```python
from build123d import *

# Parameters (mm, degrees)
BOSS_EXTRUDE1_DEPTH              = 320.675
BOSS_EXTRUDE1_DEPTH_BACK         = 320.675
SKETCH3_W                        = 50.8
SKETCH3_H                        = 25.4
SKETCH3_W_2                      = 44.45
SKETCH3_H_2                      = 19.05
CUT_EXTRUDE1_DEPTH               = 323.680609311
CUT_EXTRUDE1_DEPTH_BACK          = 323.680609311
SKETCH8_R                        = 14.2875
CUT_EXTRUDE2_DEPTH               = 323.680609311
F_10_CLEARANCE_HOLE1_D           = 4.9784
F_10_CLEARANCE_HOLE1_DEPTH       = 5.08
F_10_CLEARANCE_HOLE1_TIP         = 1.495662253
F_10_CLEARANCE_HOLE2_D           = 4.9784
F_10_CLEARANCE_HOLE3_D           = 4.9784
TAP_DRILL_FOR_8_32_TAP1_D        = 3.4544
F_10_CLEARANCE_HOLE4_AT_2_COUNT  = 2
F_10_CLEARANCE_HOLE4_AT_2_PITCH  = 21.6408
F_10_CLEARANCE_HOLE4_AT_3_COUNT  = 2
F_10_CLEARANCE_HOLE4_AT_3_PITCH  = 32.224022105
F_10_CLEARANCE_HOLE4_AT_4_COUNT  = 2
F_10_CLEARANCE_HOLE4_AT_4_PITCH  = 23.876
F_10_CLEARANCE_HOLE4_AT_5_COUNT  = 2
F_10_CLEARANCE_HOLE4_AT_5_PITCH  = 245.0465
F_10_CLEARANCE_HOLE4_AT_6_COUNT  = 2
F_10_CLEARANCE_HOLE4_AT_6_PITCH  = 246.000226396
F_10_CLEARANCE_HOLE4_AT_7_COUNT  = 2
F_10_CLEARANCE_HOLE4_AT_7_PITCH  = 268.9225
F_10_CLEARANCE_HOLE4_AT_8_COUNT  = 2
F_10_CLEARANCE_HOLE4_AT_8_PITCH  = 269.79183685
F_10_0_1935_DIAMETER_HOLE1_D     = 4.9149
F_10_0_1935_DIAMETER_HOLE1_DEPTH = 3.302
F_10_0_1935_DIAMETER_HOLE1_TIP   = 1.476584928
CUT_EXTRUDE3_DEPTH               = 323.680609311


with BuildPart() as part:
    # Sketch3 → Boss-Extrude1 (new, two sides: drawn at the far end of the back side and taken through both)
    with BuildSketch(Plane.XY.offset(-BOSS_EXTRUDE1_DEPTH_BACK)):
        Rectangle(SKETCH3_W, SKETCH3_H)
        Rectangle(SKETCH3_W_2, SKETCH3_H_2, mode=Mode.SUBTRACT)
    extrude(amount=BOSS_EXTRUDE1_DEPTH + BOSS_EXTRUDE1_DEPTH_BACK)

    # Sketch4 → Cut-Extrude1 (cut, two sides: drawn at the far end of the back side and taken through both)
    with BuildSketch(Plane(origin=(0, 12.7, 0), x_dir=(1, 0, 0), z_dir=(0, 1, 0)).offset(-CUT_EXTRUDE1_DEPTH_BACK)):
        Polygon((1322.117470931, -320.675), (25.4, -320.675), (-25.4, -320.675), (25.4, -305.627354456), (1268.718301677, 62.660305034), (3837.350959621, 420.474595165), (3890.750128875, 37.139290131), align=None)
    extrude(amount=CUT_EXTRUDE1_DEPTH + CUT_EXTRUDE1_DEPTH_BACK, mode=Mode.SUBTRACT)

    # Sketch8 → Cut-Extrude2 (cut, through all)
    with BuildSketch(Plane(origin=(0, 12.7, 0), x_dir=(1, 0, 0), z_dir=(0, 1, 0))):
        with Locations(Location((0, 266.954, 0), (0, 0, 180))):
            Circle(SKETCH8_R)
    extrude(amount=-CUT_EXTRUDE2_DEPTH, mode=Mode.SUBTRACT)

    # #10 Clearance Hole1
    with Locations(Plane(origin=(0, 12.7, 0), x_dir=(1, 0, 0), z_dir=(0, 1, 0))):
        with Locations((-12.7762, -284.753033923), (12.6238, -284.753033923), (12.6238, -301.263033923), (-12.7762, -301.263033923)):
            Hole(F_10_CLEARANCE_HOLE1_D / 2, depth=F_10_CLEARANCE_HOLE1_DEPTH)
            with Locations((0, 0, -(F_10_CLEARANCE_HOLE1_DEPTH + F_10_CLEARANCE_HOLE1_TIP / 2))):  # 118° drill point
                Cone(0, F_10_CLEARANCE_HOLE1_D / 2, F_10_CLEARANCE_HOLE1_TIP, mode=Mode.SUBTRACT)

    # #10 Clearance Hole2 (through all)
    with Locations(Plane(origin=(25.4, 0, 0), x_dir=(0, 0, -1), z_dir=(1, 0, 0))):
        with Locations((3.429, -6.35), (28.829, -6.35), (54.229, -6.35), (79.629, -6.35), (105.029, -6.35), (-288.925, -6.35), (-263.525, -6.35), (-238.126133061, -6.35)):
            Hole(F_10_CLEARANCE_HOLE2_D / 2)

    # #10 Clearance Hole3 (through all)
    with Locations(Plane(origin=(25.4, 0, 0), x_dir=(0, 0, -1), z_dir=(1, 0, 0))):
        with Locations((295.275, -6.388229415), (314.325, -6.35)):
            Hole(F_10_CLEARANCE_HOLE3_D / 2)

    # Tap Drill for #8-32 Tap1 (through all)
    with Locations(Plane(origin=(0, -12.7, 0), x_dir=(-1, 0, 0), z_dir=(0, -1, 0))):
        with Locations((-12.751963692, 254.202036308)):
            Hole(TAP_DRILL_FOR_8_32_TAP1_D / 2)

    # Sketch21 → #10 Clearance Hole4 (revolve, cut)
    with BuildSketch(Plane(origin=(11.845144988, -12.7, 30.44825), x_dir=(0, 0, -1), z_dir=(1, 0, 0))):
        Polygon((0, 0), (0, 25.4), (5.2197, 25.4), (2.4892, 22.258919064), (2.4892, 0), align=None)
    f_10_clearance_hole4 = revolve(axis=Axis((11.845144988, -19.05, 30.44825), (0, 1, 0)), mode=Mode.SUBTRACT)

    # #10 Clearance Hole4 at 2: #10 Clearance Hole4 ×2
    with Locations(*[(-i * F_10_CLEARANCE_HOLE4_AT_2_PITCH, 0, 0) for i in range(1, F_10_CLEARANCE_HOLE4_AT_2_COUNT)]):
        add(f_10_clearance_hole4, mode=Mode.SUBTRACT)

    # #10 Clearance Hole4 at 3: #10 Clearance Hole4 ×2
    with Locations(*[Vector(-0.6715735214342001, 0, 0.7409379227090944) * (i * F_10_CLEARANCE_HOLE4_AT_3_PITCH) for i in range(1, F_10_CLEARANCE_HOLE4_AT_3_COUNT)]):
        add(f_10_clearance_hole4, mode=Mode.SUBTRACT)

    # #10 Clearance Hole4 at 4: #10 Clearance Hole4 ×2
    with Locations(*[(0, 0, i * F_10_CLEARANCE_HOLE4_AT_4_PITCH) for i in range(1, F_10_CLEARANCE_HOLE4_AT_4_COUNT)]):
        add(f_10_clearance_hole4, mode=Mode.SUBTRACT)

    # #10 Clearance Hole4 at 5: #10 Clearance Hole4 ×2
    with Locations(*[(0, 0, -i * F_10_CLEARANCE_HOLE4_AT_5_PITCH) for i in range(1, F_10_CLEARANCE_HOLE4_AT_5_COUNT)]):
        add(f_10_clearance_hole4, mode=Mode.SUBTRACT)

    # #10 Clearance Hole4 at 6: #10 Clearance Hole4 ×2
    with Locations(*[Vector(-0.08797065074713521, 0, -0.9961230669988149) * (i * F_10_CLEARANCE_HOLE4_AT_6_PITCH) for i in range(1, F_10_CLEARANCE_HOLE4_AT_6_COUNT)]):
        add(f_10_clearance_hole4, mode=Mode.SUBTRACT)

    # #10 Clearance Hole4 at 7: #10 Clearance Hole4 ×2
    with Locations(*[(0, 0, -i * F_10_CLEARANCE_HOLE4_AT_7_PITCH) for i in range(1, F_10_CLEARANCE_HOLE4_AT_7_COUNT)]):
        add(f_10_clearance_hole4, mode=Mode.SUBTRACT)

    # #10 Clearance Hole4 at 8: #10 Clearance Hole4 ×2
    with Locations(*[Vector(-0.08021295326304817, 0, -0.9967777496156403) * (i * F_10_CLEARANCE_HOLE4_AT_8_PITCH) for i in range(1, F_10_CLEARANCE_HOLE4_AT_8_COUNT)]):
        add(f_10_clearance_hole4, mode=Mode.SUBTRACT)

    # #10 (0.1935) Diameter Hole1
    with Locations(Plane(origin=(25.4, 0, 0), x_dir=(0, 0, -1), z_dir=(1, 0, 0))):
        with Locations((269.875, -6.35)):
            Hole(F_10_0_1935_DIAMETER_HOLE1_D / 2, depth=F_10_0_1935_DIAMETER_HOLE1_DEPTH)
            with Locations((0, 0, -(F_10_0_1935_DIAMETER_HOLE1_DEPTH + F_10_0_1935_DIAMETER_HOLE1_TIP / 2))):  # 118° drill point
                Cone(0, F_10_0_1935_DIAMETER_HOLE1_D / 2, F_10_0_1935_DIAMETER_HOLE1_TIP, mode=Mode.SUBTRACT)

    # Sketch24 → Cut-Extrude3 (cut, through all)
    with BuildSketch(Plane.XZ.offset(12.7)):
        with BuildLine():
            Line((-5.356640498, 314.737886431), (-17.533651131, 318.344881309))
            Line((-17.533651131, 318.344881309), (-18.255050107, 315.909479182))
            ThreePointArc((-18.255050107, 315.909479182), (-13.970042229, 308.017476427), (-6.078039474, 312.302484305))
            Line((-6.078039474, 312.302484305), (-5.356640498, 314.737886431))
        make_face()
    extrude(amount=-CUT_EXTRUDE3_DEPTH, mode=Mode.SUBTRACT)


solid = part.part
```
Read the model definition and answer for the solid it produces. Units are mm, in the model's axes. A direction names the side the tool comes from. Coordinates: 2 decimals unless noted, no trailing zeros. Loops run counter-clockwise (first coordinate to the right, second up) from the corner with the lowest first, then second, coordinate; pieces in that order, holes last. Notation, with made-up numbers: (87.25, 35.25) -> (105.25, 35.25) arc R13 ccw to (105.25, 43.25) -> close; hole circle Ø4 at (8.25, -32). An arc over 180 degrees is marked (long way). Return JSON: item names as keys, results as strings.
Item 1: Find the intervals of material crossed by probe 1 along Y at (x, z) = (19.5, 72) (3 decimals); probe 2 along X at (y, z) = (-8.5, -187.5) (3 decimals); probe 3 along Z at (x, y) = (22.5, 3) (3 decimals), in increasing order.
Answers:
{"probe 1": "y = -12.7 to -9.525, 9.525 to 12.7", "probe 2": "x = -25.4 to -22.225, 22.225 to 25.4", "probe 3": "z = -320.675 to 306.486"}
Item 2: For a pull along Y with two mould halves and no side action, classify faces 3 (the flat face through (0, 10, -320.675)), 4 (the flat face through (-22.225, 0, -5)), 5 (the conical face through (-8.2, 9.71, 56.4)) as +Y half, -Y half, draft (parallel to the pull), parting line (faces both ways), or undercut.
Answers:
{"face 3": "draft", "face 4": "undercut", "face 5": "+Y half"}
Item 3: For faces 1 (the flat face through (25.4, 0, -12)), 2 (the flat face through (0, -9.525, -5)), determine the directions among +Z, -Z, +X, -X, +Y, -Y from which every point of the face is accessible in a straight line to the end or side of a thin tool.
Answers:
{"face 1": "+Z, -Z, +X, +Y, -Y", "face 2": "+Z, -Z"}
Item 4: Find section B-B (z = -181). Determine the outline of the cut face in (x, y) (3 decimals).
Answers:
{"outline": "(-25.4, -12.7) -> (25.4, -12.7) -> (25.4, 12.7) -> (-25.4, 12.7) -> close; hole (-22.225, -9.525) -> (22.225, -9.525) -> (22.225, 9.525) -> (-22.225, 9.525) -> close"}
Item 5: Flat-ended cylindrical pins translate along their axes: P1, Ø8, axis at x = 11.85, z = 30.45, coming from the -Y side; P2, Ø4, axis at x = -9.8, z = -214.6, coming from the -Y side; P3, Ø8, axis at x = -9.8, z = 54.32, coming from the +Y side. Find the tip coordinate at first contact, or state that the pin passes through.
Answers:
{"P1": "stops at y = -12.7", "P2": "passes through", "P3": "stops at y = 11.3"}
Item 6: Find section A-A (y = 1). Determine the outline of the cut face in (x, z) (3 decimals).
Answers:
{"outline": "(-25.4, -320.675) -> (-22.225, -320.675) -> (-22.225, 319.735) -> (-25.4, 320.675) -> close; (22.225, -320.675) -> (25.4, -320.675) -> (25.4, 305.627) -> (22.225, 306.568) -> close"}
